Part model, mm, in its own coordinate system. A direction names the side the tool comes from. Give positions to 0.01 mm unless a question says otherwise; leave off trailing zeros. Write each loop counter-clockwise with the first axis right and the second up, starting at its lowest first coordinate (ties: lowest second). Pieces come first, ordered by that corner, then holes.
```python
from build123d import *

# Parameters (mm, degrees)
SKETCH3_R               = 3
CUT_EXTRUDE1_DEPTH      = 6
CUT_EXTRUDE1_DEPTH_BACK = 6


with BuildPart() as part:
    # Sweep1: sweep along a path in Sketch1
    with BuildLine(Plane(origin=(0, 0, 0), x_dir=(1, 0, 0), z_dir=(0, 1, 0))) as sweep1_path:
        Line((0, 100), (0, 0))
        Line((0, 0), (100, 0))
    # Sketch2 → Sweep1 (sweep)
    with BuildSketch(Plane.XY.offset(-100)):
        Polygon((5.773502692, 0), (2.886751346, 5), (-2.886751346, 5), (-5.773502692, 0), (-2.886751346, -5), (2.886751346, -5), align=None)
    sweep(path=sweep1_path.line, transition=Transition.RIGHT)

    # Sketch3 → Cut-Extrude1 (cut, two sides)
    with BuildSketch(Plane(origin=(0, 0, 0), x_dir=(1, 0, 0), z_dir=(0, 1, 0))) as cut_extrude1_sk:
        with Locations((0, 90)):
            Circle(SKETCH3_R)
        with Locations((90, 0)):
            Circle(SKETCH3_R)
    extrude(amount=CUT_EXTRUDE1_DEPTH, mode=Mode.SUBTRACT)
    extrude(cut_extrude1_sk.sketch, amount=-CUT_EXTRUDE1_DEPTH_BACK, mode=Mode.SUBTRACT)


solid = part.part
```
1) Pin check, flat tips, straight feed: pin 1 Ø1.5 at (y, z) = (-4, -48) entering from -X; pin 2 Ø4 at (y, z) = (3, -62) entering from -X. Stop position of each tip, or through.
Answers follow:
pin 1: stops at x = -3.9
pin 2: stops at x = -5.2
2) Saw through at C-C, the plane z = -15. Write the cut outline in (x, y).
Answers follow:
outline: (-5.77, 0) - (-2.89, -5) - (2.89, -5) - (5.77, 0) - (2.89, 5) - (-2.89, 5) - close
3) Saw through at B-B, the plane x = 0. Write the cut outline in (y, z).
Answers follow:
outline: (-5, -100) - (5, -100) - (5, -93) - (-5, -93) - close; (-5, -87) - (5, -87) - (5, 2.89) - (0, 5.77) - (-5, 2.89) - close
4) 3-axis set-ups, long thin cutter, end or side, ignore diameter. For faces 1 (the face through (4.31, -2.535, -50.764)), 2 (the face through (-4.31, 2.535, -46.373)), 3 (the face through (4.35, 2.465, -50.764)): which of +Z, -Z, +X, -X, +Y, -Y reach the whole face in a straight line?
Answers follow:
face 1: -Z, +X, -Y
face 2: +Z, -Z, -X, +Y
face 3: -Z, +X, +Y
5) Saw through at A-A, the plane z = 0. Write the cut outline in (x, y), then the cut area to 3 significant figures.
Answers follow:
outline: (-5.77, 0) - (-2.89, -5) - (87, -5) - (87, 5) - (-2.89, 5) - close; (93, -5) - (100, -5) - (100, 5) - (93, 5) - close
area: 983 mm2
6) Saw through at D-D, the plane x = 31.5. Write the cut outline in (y, z).
Answers follow:
outline: (-5, -2.89) - (0, -5.77) - (5, -2.89) - (5, 2.89) - (0, 5.77) - (-5, 2.89) - close
7) Wall check: L1, parallel to Z at x = 0, y = 1.55; L2, parallel to Z at x = 90, y = 2.9; L3, parallel to X at y = 3.4, z = -90. Give the ranges that are in metal, low to high.
Answers follow:
L1: z = -100 to -93, -87 to 4.88
L2: z = -4.1 to -3, 3 to 4.1
L3: x = -3.81 to -3, 3 to 3.81
